Model file for the job. Use its own axes, mm. Coordinates: 2 decimals unless noted, no trailing zeros. Order: outer loops, then holes, each group sorted by start corner. A loop starts at its lowest first (then second) coordinate and runs counter-clockwise, first axis right, second up. Notation, with made-up numbers: (35, 67) -> (62, 67) arc R16 cw to (62, 76) -> close; hole circle Ø2 at (58.5, 50.5). An arc over 180 degrees is marked (long way). Use CSV: the item, a comma, the result in double quotes. Start each with the question number.
(1) Cut at A-A on x = 17. Write the cut outline in (y, z) (3 decimals).
(2) Cut at B-B on y = 25.5. Write the cut outline in (x, z) (3 decimals).
(3) Probe L1, parallel to Y at x = 15, z = 2.7; L2, parallel to Y at x = -37.5, z = 0.85; L3, parallel to X at y = 44.5, z = 2.15. List the from-to ranges inside material, lowest first.
(4) Cut at D-D on y = 42. Write the cut outline in (x, z) (3 decimals), plus the area to 3 significant figures.
(5) Cut at C-C on x = -20.5. Write the cut outline in (y, z) (3 decimals), plus the area to 3 significant figures.
```python
from build123d import *

# Parameters (mm, degrees)
F0_W     = 83.5
F0_H     = 65.2625
F0_W_2   = 8
F0_H_2   = 3.175
F0_W_3   = 77.5
F0_H_3   = 29.325
F0_W_4   = 34.5
F0_H_4   = 20.675
F0_W_5   = 6
F0_W_6   = 10
F0_H_5   = 10
F0_R     = 1.2
F1_DEPTH = 3.175


# Not quite as in the source:
# - a length typed as a fraction of an inch, garbled in the dataset ("3 / 203.2 mm" for 3/8 in), is restored
# - a feature names something its author has since deleted; it is built from what else it names


with BuildPart() as f1:
    # F0 (on Top) → F1 (new body)
    with BuildSketch(Plane.XY):
        with Locations((-5.970182175, 24.7772044539)):
            Rectangle(F0_W, F0_H)
        with Locations((-20.970182175, -3.1790455461)):
            Rectangle(F0_W_2, F0_H_2, mode=Mode.SUBTRACT)
        with BuildLine():
            ThreePointArc((-9.470182175, -4.6790455461), (-10.5308423468, -2.1183853743), (-7.970182175, -3.1790455461))
            ThreePointArc((-7.970182175, -3.1790455461), (-8.4095220032, -4.2397057179), (-9.470182175, -4.6790455461))
        make_face(mode=Mode.SUBTRACT)
        with Locations((2.029817825, -3.1790455461)):
            Rectangle(F0_W_2, F0_H_2, mode=Mode.SUBTRACT)
        with Locations((-5.970182175, 16.0709544539)):
            Rectangle(F0_W_3, F0_H_3, mode=Mode.SUBTRACT)
        Polygon((-44.720182175, 34.4084544539), (-44.720182175, 44.4084544539), (-44.720182175, 54.4084544539), (-34.720182175, 54.4084544539), (-34.720182175, 44.4084544539), (-34.720182175, 34.4084544539), align=None, mode=Mode.SUBTRACT)
        with Locations((-14.470182175, 44.0709544539)):
            Rectangle(F0_W_4, F0_H_4, mode=Mode.SUBTRACT)
        with Locations((12.779817825, 35.3209544539)):
            Rectangle(F0_W_5, F0_H_2, mode=Mode.SUBTRACT)
        with BuildLine():
            ThreePointArc((21.279817825, 33.8209544539), (20.2191576532, 36.3816146257), (22.779817825, 35.3209544539))
            ThreePointArc((22.779817825, 35.3209544539), (22.3404779968, 34.2602942821), (21.279817825, 33.8209544539))
        make_face(mode=Mode.SUBTRACT)
        with Locations((29.779817825, 35.3209544539)):
            Rectangle(F0_W_5, F0_H_2, mode=Mode.SUBTRACT)
        Polygon((25.779817825, 44.4084544539), (15.779817825, 44.4084544539), (5.779817825, 44.4084544539), (5.779817825, 54.4084544539), (15.779817825, 54.4084544539), (25.779817825, 54.4084544539), align=None, mode=Mode.SUBTRACT)
        with Locations((-39.720182175, 39.4084544539)):
            Rectangle(F0_W_6, F0_H_5)
        with Locations((-39.720182175, 39.4084544539)):
            Circle(F0_R, mode=Mode.SUBTRACT)
        with Locations((10.779817825, 49.4084544539)):
            Rectangle(F0_W_6, F0_H_5)
        with Locations((10.779817825, 49.4084544539)):
            Circle(F0_R, mode=Mode.SUBTRACT)
    extrude(amount=F1_DEPTH)


solid = f1.part
```
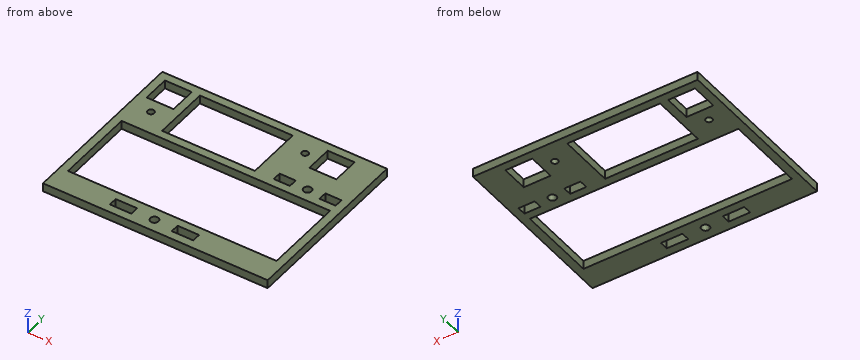
Outcome:
1,outline,"(-7.854, 0) -> (1.408, 0) -> (1.408, 3.175) -> (-7.854, 3.175) -> close; (30.733, 0) -> (44.408, 0) -> (44.408, 3.175) -> (30.733, 3.175) -> close; (54.408, 0) -> (57.408, 0) -> (57.408, 3.175) -> (54.408, 3.175) -> close"
2,outline,"(-47.72, 0) -> (-44.72, 0) -> (-44.72, 3.175) -> (-47.72, 3.175) -> close; (32.78, 0) -> (35.78, 0) -> (35.78, 3.175) -> (32.78, 3.175) -> close"
3,L1,"-7.85 to 1.41, 30.73 to 33.73, 36.91 to 57.41"
3,L2,"-7.85 to 1.41, 30.73 to 44.41, 54.41 to 57.41"
3,L3,"-47.72 to -44.72, -34.72 to -31.72, 2.78 to 15.78, 25.78 to 35.78"
4,outline,"(-47.72, 0) -> (-31.72, 0) -> (-31.72, 3.175) -> (-47.72, 3.175) -> close; (2.78, 0) -> (35.78, 0) -> (35.78, 3.175) -> (2.78, 3.175) -> close"
4,area,"156 mm2"
5,outline,"(-7.854, 0) -> (-4.767, 0) -> (-4.767, 3.175) -> (-7.854, 3.175) -> close; (-1.592, 0) -> (1.408, 0) -> (1.408, 3.175) -> (-1.592, 3.175) -> close; (30.733, 0) -> (33.733, 0) -> (33.733, 3.175) -> (30.733, 3.175) -> close; (54.408, 0) -> (57.408, 0) -> (57.408, 3.175) -> (54.408, 3.175) -> close"
5,area,"38.4 mm2"
